CAD build for the part. Positions are in the model's coordinates, mm. Face numbers are marked on the shaded views. A direction names the side the tool comes from. Coordinates: 2 decimals unless noted, no trailing zeros. Write each loop counter-clockwise with the first axis right and the second up, starting at its lowest first coordinate (ties: lowest second). Pieces come first, ordered by that corner, then holes. Notation, with made-up numbers: (2, 59.25) - (9, 59.25) arc R11 ccw to (9, 63.25) - close; hole circle Ø1 at (-20, -8). An arc over 180 degrees is marked (long way). Answer in a Markdown table with one row per item. Add a question column.
Q1. Band-saw the part on B-B (z = 6.5). List the corners of the cut face in (x, y), and give its area (3 significant figures).
Q2. Band-saw the part on C-C (x = 6.75). List the corners of the cut face in (y, z), and give its area (3 significant figures).
Q3. Two-plate mould, pull along X, no slides. Class the marked faces 3, 4, 5 and 6: +X half, -X half, draft (parallel to the pull), parting line (faces both ways), or undercut.
Q4. Band-saw the part on D-D (y = 4). List the corners of the cut face in (x, z), and give its area (3 significant figures).
Q5. 3-axis set-ups, long thin cutter, end or side, ignore diameter. For the marked faces 1 and 2: which of +Z, -Z, +X, -X, +Y, -Y reach the whole face in a straight line?
Q6. Drill centre lines: line 1 along Z through (x, y) = (-6.75, 0); line 2 along Y through (x, z) = (0, 18); line 3 along Z through (x, y) = (-8.5, 0). Where is each one in solid material? Low to high. Write a range as from..to.
Q7. Pin check, flat tips, straight feed: pin 1 (3 mm diameter, centred on y = 4.5, z = 23.5, fed in from +X); pin 2 (2 mm diameter, centred on x = 8, y = 5, fed in from -Z); pin 3 (10 mm diameter, centred on x = -9.5, z = 39, fed in from +Y). Stop position of each tip, or through.
Q8. Band-saw the part on A-A (y = 0). List the corners of the cut face in (x, z).
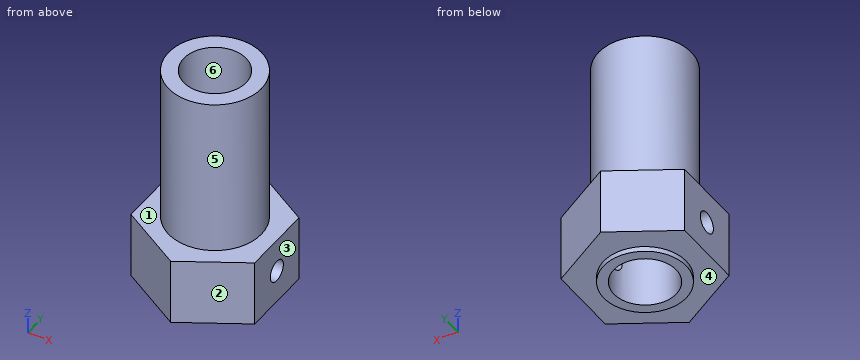
```python
from build123d import *

# Parameters (mm, degrees)
EXTRUDE_1_DEPTH     = 13
SKETCH_2_R          = 9
EXTRUDE_2_DEPTH     = 31
SKETCH_3_R          = 8
EXTRUDE_3_DEPTH     = 1
SKETCH_4_R          = 6.05
CUT_EXTRUDE_1_DEPTH = 45
SKETCH_5_R          = 2.05
CUT_EXTRUDE_2_DEPTH = 25


with BuildPart() as part:
    # 草图1 → 凸台-拉伸1 (new body)
    with BuildSketch(Plane.XY):
        Polygon((0, 13.856406461), (-12, 6.92820323), (-12, -6.92820323), (0, -13.856406461), (12, -6.92820323), (12, 6.92820323), align=None)
    extrude(amount=EXTRUDE_1_DEPTH)

    # 草图2 → 凸台-拉伸2 (add)
    with BuildSketch(Plane.XY.offset(13)):
        Circle(SKETCH_2_R)
    extrude(amount=EXTRUDE_2_DEPTH)

    # 草图3 → 凸台-拉伸3 (add)
    with BuildSketch(Plane(origin=(0, 0, 0), x_dir=(-1, 0, 0), z_dir=(0, 0, -1))):
        Circle(SKETCH_3_R)
    extrude(amount=EXTRUDE_3_DEPTH)

    # 草图4 → 切除-拉伸1 (cut)
    with BuildSketch(Plane(origin=(0, 0, -1), x_dir=(-1, 0, 0), z_dir=(0, 0, -1))):
        Circle(SKETCH_4_R)
    extrude(amount=-CUT_EXTRUDE_1_DEPTH, mode=Mode.SUBTRACT)

    # 草图5 → 切除-拉伸2 (cut, symmetric)
    with BuildSketch(Plane(origin=(0, 0, 0), x_dir=(0, 0, -1), z_dir=(1, 0, 0))):
        with Locations((-6.5, 0)):
            Circle(SKETCH_5_R)
    extrude(amount=CUT_EXTRUDE_2_DEPTH, both=True, mode=Mode.SUBTRACT)


solid = part.part
```
Checked values:
| question | item | result |
|---|---|---|
| 1 | outline | (-12, -6.93) - (0, -13.86) - (12, -6.93) - (12, -2.05) - (5.69, -2.05) arc R6.05 cw to (-5.69, -2.05) - (-12, -2.05) - close; (-12, 2.05) - (-5.69, 2.05) arc R6.05 cw to (5.69, 2.05) - (12, 2.05) - (12, 6.93) - (0, 13.86) - (-12, 6.93) - close |
| 1 | area | 334 mm² |
| 2 | outline | (-9.96, 0) - (-4.29, 0) - (-4.29, -1) - (4.29, -1) - (4.29, 0) - (9.96, 0) - (9.96, 13) - (5.95, 13) - (5.95, 44) - (-5.95, 44) - (-5.95, 13) - (-9.96, 13) - close; hole circle Ø4.1 at (0, 6.5) |
| 2 | area | 623 mm² |
| 3 | face 3 | +X half |
| 3 | face 4 | draft |
| 3 | face 5 | parting line |
| 3 | face 6 | undercut |
| 4 | outline | (-12, 0) - (-6.93, 0) - (-6.93, -1) - (-4.54, -1) - (-4.54, 44) - (-8.06, 44) - (-8.06, 13) - (-12, 13) - close; (4.54, -1) - (6.93, -1) - (6.93, 0) - (12, 0) - (12, 13) - (8.06, 13) - (8.06, 44) - (4.54, 44) - close |
| 4 | area | 417 mm² |
| 5 | face 1 | +Z |
| 5 | face 2 | +Z, -Z, +X, -Y |
| 6 | line 1 | z = -1..4.45, 8.55..44 |
| 6 | line 2 | y = -9..-6.05, 6.05..9 |
| 6 | line 3 | z = 0..4.45, 8.55..44 |
| 7 | pin 1 | stops at x = 8.49 |
| 7 | pin 2 | stops at z = 0 |
| 7 | pin 3 | stops at y = 7.79 |
| 8 | outline | (-12, 0) - (-8, 0) - (-8, -1) - (-6.05, -1) - (-6.05, 4.45) - (-12, 4.45) - close; (-12, 8.55) - (-6.05, 8.55) - (-6.05, 44) - (-9, 44) - (-9, 13) - (-12, 13) - close; (6.05, -1) - (8, -1) - (8, 0) - (12, 0) - (12, 4.45) - (6.05, 4.45) - close; (6.05, 8.55) - (12, 8.55) - (12, 13) - (9, 13) - (9, 44) - (6.05, 44) - close |
